from build123d import *

# Parameters (mm, degrees)
SKETCH1_W           = 150
SKETCH1_H           = 200
BOSS_EXTRUDE1_DEPTH = 100
SHELL2_T            = -5
SKETCH5_R           = 1.9
CUT_EXTRUDE2_DEPTH  = 10
BOSS_EXTRUDE4_DEPTH = 200
SKETCH9_W           = 101.133931545
SKETCH9_H           = 31.996148617
CUT_EXTRUDE4_DEPTH  = 236.849528301
SKETCH10_R          = 4
CUT_EXTRUDE5_DEPTH  = 10
CUT_EXTRUDE7_REACH  = 162.078
SKETCH11_W          = 140
SKETCH11_H          = 5
SKETCH15_R          = 1.2
CUT_EXTRUDE11_DEPTH = 10
SKETCH36_W          = 60
SKETCH36_H          = 5
BOSS_EXTRUDE7_DEPTH = 10
SKETCH37_R          = 3.5
CUT_EXTRUDE15_DEPTH = 60
SKETCH38_R          = 5
CUT_EXTRUDE16_DEPTH = 70
SKETCH42_W          = 159.84088679
SKETCH42_H          = 73
CUT_EXTRUDE20_DEPTH = 236.849528301


with BuildPart() as part:
    # Sketch1 → Boss-Extrude1 (new body)
    with BuildSketch(Plane(origin=(0, 0, 0), x_dir=(1, 0, 0), z_dir=(0, 1, 0))):
        Rectangle(SKETCH1_W, SKETCH1_H)
    extrude(amount=BOSS_EXTRUDE1_DEPTH)

    # Shell2
    shell2_openings = [part.faces().sort_by_distance(p)[0] for p in [
        (0, 50, -100),
        (0, 50, 100),
    ]]
    offset(amount=SHELL2_T, openings=shell2_openings, kind=Kind.INTERSECTION)

    # Sketch5 → Cut-Extrude2 (cut)
    with BuildSketch(Plane.XZ):
        with Locations(Location((-65, 91, 0), (0, 0, 270))):
            Circle(SKETCH5_R)
        with Locations(Location((-35, 91, 0), (0, 0, 270))):
            Circle(SKETCH5_R)
        with Locations(Location((-65, 67, 0), (0, 0, 270))):
            Circle(SKETCH5_R)
        with Locations(Location((-35, 67, 0), (0, 0, 270))):
            Circle(SKETCH5_R)
    cut_extrude2 = extrude(amount=-CUT_EXTRUDE2_DEPTH, mode=Mode.SUBTRACT)

    # Mirror2: Cut-Extrude2 across plane
    add(cut_extrude2.mirror(Plane.XY), mode=Mode.SUBTRACT)

    # Sketch8 → Boss-Extrude4 (add, through all)
    with BuildSketch(Plane.XY.offset(100)):
        Polygon((-15, 17), (75, 17), (75, 22), (-20, 22), (-20, 0), (-15, 0), align=None)
    extrude(amount=-BOSS_EXTRUDE4_DEPTH)

    # Sketch9 → Cut-Extrude4 (cut, through all)
    with BuildSketch(Plane.XY.offset(100)):
        with Locations((35.566965773, 1.001925691)):
            Rectangle(SKETCH9_W, SKETCH9_H)
    extrude(amount=-CUT_EXTRUDE4_DEPTH, mode=Mode.SUBTRACT)

    # Sketch10 → Cut-Extrude5 (cut)
    with BuildSketch(Plane.XZ.offset(-17)):
        with Locations((60, 0)):
            Circle(SKETCH10_R)
    extrude(amount=-CUT_EXTRUDE5_DEPTH, mode=Mode.SUBTRACT)

    # Cut-Extrude7: up to this face of the body (flat: up to its plane)
    cut_extrude7_end = Plane(part.part.faces().sort_by_distance((-44.954220044, 5, 0))[0])
    # Sketch11 → Cut-Extrude7 (cut, up to the picked face)
    with BuildSketch(Plane(origin=(0, 100, 0), x_dir=(1, 0, 0), z_dir=(0, 1, 0)), mode=Mode.PRIVATE) as cut_extrude7_sk1:
        with Locations((0, -92.5)):
            Rectangle(SKETCH11_W, SKETCH11_H)
    cut_extrude7_tool1 = split(extrude(cut_extrude7_sk1.sketch, amount=-CUT_EXTRUDE7_REACH, mode=Mode.PRIVATE), bisect_by=cut_extrude7_end, keep=Keep.BOTH, mode=Mode.PRIVATE)
    cut_extrude7 = cut_extrude7_tool1.solids().sort_by(Axis((0, 100, 92.5), (0, -1, 0)))[0]
    add(cut_extrude7, mode=Mode.SUBTRACT)

    # Mirror3: Cut-Extrude7 across plane
    add(cut_extrude7.mirror(Plane.XY), mode=Mode.SUBTRACT)

    # Sketch15 → Cut-Extrude11 (cut)
    with BuildSketch(Plane(origin=(0, 100, 0), x_dir=(1, 0, 0), z_dir=(0, 1, 0))):
        with Locations(Location((50, 28, 0), (0, 0, 270))):
            Circle(SKETCH15_R)
        with Locations(Location((50, -28, 0), (0, 0, 270))):
            Circle(SKETCH15_R)
        with Locations(Location((-20, 20, 0), (0, 0, 270))):
            Circle(SKETCH15_R)
        with Locations(Location((-20, -20, 0), (0, 0, 270))):
            Circle(SKETCH15_R)
    extrude(amount=-CUT_EXTRUDE11_DEPTH, mode=Mode.SUBTRACT)

    # Sketch36 → Boss-Extrude7 (add)
    with BuildSketch(Plane.ZY.offset(-70)):
        with Locations((-13.202053215, 62.5)):
            Rectangle(SKETCH36_W, SKETCH36_H)
    boss_extrude7 = extrude(amount=BOSS_EXTRUDE7_DEPTH)

    # Mirror5: Boss-Extrude7 across plane
    add(boss_extrude7.mirror(Plane(origin=(0, 0, 0), x_dir=(0, 0, 1), z_dir=(1, 0, 0))))

    # Sketch37 → Cut-Extrude15 (cut)
    with BuildSketch(Plane(origin=(75, 0, 0), x_dir=(0, 0, -1), z_dir=(1, 0, 0))):
        with Locations((0, 75)):
            Circle(SKETCH37_R)
    extrude(amount=-CUT_EXTRUDE15_DEPTH, mode=Mode.SUBTRACT)

    # Sketch38 → Cut-Extrude16 (cut)
    with BuildSketch(Plane.ZY.offset(75)):
        with Locations((0, 80)):
            Circle(SKETCH38_R)
    extrude(amount=-CUT_EXTRUDE16_DEPTH, mode=Mode.SUBTRACT)

    # Sketch42 → Cut-Extrude20 (cut, through all)
    with BuildSketch(Plane.XY.offset(100)):
        with Locations((-9.920443395, 58.5)):
            Rectangle(SKETCH42_W, SKETCH42_H)
        Polygon((-89.84088679, 95), (70, 95), (99.534009441, 95), (99.534009441, 106.078306858), (-89.84088679, 106.078306858), align=None)
        Polygon((106.355095751, 22), (70, 22), (-89.84088679, 22), (-89.84088679, -3.777083183), (106.355095751, -3.777083183), align=None)
    extrude(amount=-CUT_EXTRUDE20_DEPTH, mode=Mode.SUBTRACT)


solid = part.part
Input: part model. Units: mm. Frame: model coordinates. Coordinates: 2 decimals unless noted, no trailing zeros. Loops run counter-clockwise (first coordinate to the right, second up) from the corner with the lowest first, then second, coordinate; pieces in that order, holes last. Notation, with made-up numbers: (40.25, 4.5) - (86.25, 4.5) arc R14 cw to (86.25, 23.5) - close; hole circle Ø9 at (-27, -15.75). An arc over 180 degrees is marked (long way). Answer in a Markdown table with one row per item. Add a question column.
Item 1: Mould query, pull axis Z, two halves, no side actions, for faces 1 (the flat face through (72, 59, -100)), 2 (the cylindrical face through (72.535, 71.583, 0.759)), 3 (the flat face through (75, 58, 1)), 4 (the flat face through (72, 59, 100)). Classes: released by +Z, released by -Z, zero draft, split by the parting line, or undercut.
Item 2: Section query B-B on y = 75. Return the cut outline in (x, z), then the cut area to 3 significant figures.
Item 3: Section query A-A on z = 0. Return the cut outline in (x, y).
Item 4: Line query: line 1 along Y through (x, z) = (71.2, 0); line 2 along Z through (x, y) = (74.4, 72.5). Output: solid intervals per line, ascending. Write a range as [from, to].
Recorded:
| question | item | result |
|---|---|---|
| 1 | face 1 | released by -Z |
| 1 | face 2 | undercut |
| 1 | face 3 | zero draft |
| 1 | face 4 | released by +Z |
| 2 | outline | (70, -100) - (75, -100) - (75, -3.5) - (70, -3.5) - close; (70, 3.5) - (75, 3.5) - (75, 100) - (70, 100) - close |
| 2 | area | 965 mm^2 |
| 3 | outline | (70, 22) - (75, 22) - (75, 71.5) - (70, 71.5) - close; (70, 78.5) - (75, 78.5) - (75, 95) - (70, 95) - close |
| 4 | line 1 | [22, 71.5], [78.5, 95] |
| 4 | line 2 | [-100, -2.45], [2.45, 100] |
